from build123d import *

# Parameters (mm, degrees)
SKETCH1_R               = 2.54
BOSS_EXTRUDE1_DEPTH     = 15.24
CUT_EXTRUDE1_DEPTH      = 28.358513503
SKETCH3_W               = 3.302
SKETCH3_H               = 15.39875
CUT_EXTRUDE2_DEPTH      = 26.630137107
CUT_EXTRUDE2_DEPTH_BACK = 26.630137107
SKETCH5_R               = 5.9055
SKETCH5_R_2             = 2.54
BOSS_EXTRUDE2_DEPTH     = 3.81
CUT_EXTRUDE3_DEPTH      = 3.81
FILLET1_R               = 1.27


with BuildPart() as part:
    # Sketch1 → Boss-Extrude1 (new body)
    with BuildSketch(Plane(origin=(0, 0, 0), x_dir=(0, 0, -1), z_dir=(1, 0, 0))):
        with BuildLine():
            Line((-6.35, 0), (-4.6736, 0))
            Line((-4.6736, 0), (-4.6736, -15.7))
            Line((-4.6736, -15.7), (-1.6256, -15.7))
            Line((-1.6256, -15.7), (-1.6256, 0))
            Line((-1.6256, 0), (1.6256, 0))
            Line((1.6256, 0), (1.6256, -15.7))
            Line((1.6256, -15.7), (4.6736, -15.7))
            Line((4.6736, -15.7), (4.6736, 0))
            Line((4.6736, 0), (6.35, 0))
            Line((6.35, 0), (6.35, 6.319735583))
            ThreePointArc((6.35, 6.319735583), (6.479041034, 7.59337978), (6.86091954, 8.815259453))
            ThreePointArc((6.86091954, 8.815259453), (0, 19.20875), (-6.86091954, 8.815259453))
            ThreePointArc((-6.86091954, 8.815259453), (-6.479041034, 7.59337978), (-6.35, 6.319735583))
            Line((-6.35, 6.319735583), (-6.35, 0))
        make_face()
        with Locations((0, 11.7475)):
            Circle(SKETCH1_R, mode=Mode.SUBTRACT)
    extrude(amount=-BOSS_EXTRUDE1_DEPTH)

    # Sketch2 → Cut-Extrude1 (cut, through all)
    with BuildSketch(Plane.XY.offset(4.6736)):
        with BuildLine():
            ThreePointArc((-5.08, -8.08), (-5.823948776, -6.283948776), (-7.62, -5.54))
            Line((-7.62, -5.54), (-7.62, -10.62))
            ThreePointArc((-7.62, -10.62), (-5.823948776, -9.876051224), (-5.08, -8.08))
        make_face()
        with BuildLine():
            Line((-7.62, -10.62), (-7.62, -5.54))
            ThreePointArc((-7.62, -5.54), (-10.16, -8.08), (-7.62, -10.62))
        make_face()
        with BuildLine():
            ThreePointArc((-7.62, -15.7), (-13.008153673, -13.468153673), (-15.24, -8.08))
            Line((-15.24, -8.08), (-15.24, -15.7))
            Line((-15.24, -15.7), (-7.62, -15.7))
        make_face()
        with BuildLine():
            Line((0, -15.7), (0, -8.08))
            ThreePointArc((0, -8.08), (-2.231846327, -13.468153673), (-7.62, -15.7))
            Line((-7.62, -15.7), (0, -15.7))
        make_face()
    extrude(amount=-CUT_EXTRUDE1_DEPTH, mode=Mode.SUBTRACT)

    # Sketch3 → Cut-Extrude2 (cut, two sides)
    with BuildSketch(Plane.XY) as cut_extrude2_sk:
        with Locations((-4.318, 11.509375)):
            Rectangle(SKETCH3_W, SKETCH3_H)
        with Locations((-10.922, 11.509375)):
            Rectangle(SKETCH3_W, SKETCH3_H)
    extrude(amount=CUT_EXTRUDE2_DEPTH, mode=Mode.SUBTRACT)
    extrude(cut_extrude2_sk.sketch, amount=-CUT_EXTRUDE2_DEPTH_BACK, mode=Mode.SUBTRACT)

    # Sketch5 → Boss-Extrude2 (add)
    with BuildSketch(Plane(origin=(0, 0, 0), x_dir=(0, 0, -1), z_dir=(1, 0, 0))):
        with Locations(Location((0, 11.7475, 0), (0, 0, 180))):
            Circle(SKETCH5_R)
        with Locations((0, 11.7475)):
            Circle(SKETCH5_R_2, mode=Mode.SUBTRACT)
    extrude(amount=BOSS_EXTRUDE2_DEPTH)

    # Sketch6 → Cut-Extrude3 (cut)
    with BuildSketch(Plane(origin=(3.81, 0, 0), x_dir=(0, 0, -1), z_dir=(1, 0, 0))):
        Polygon((0, 16.322885413), (-3.9624, 14.035192707), (-3.9624, 9.459807293), (0, 7.172114587), (3.9624, 9.459807293), (3.9624, 14.035192707), align=None)
    extrude(amount=-CUT_EXTRUDE3_DEPTH, mode=Mode.SUBTRACT)

    # Fillet1
    fillet1_edges = [part.edges().sort_by_distance(p)[0] for p in [
        (0, 11.7475, -5.9055),
        (3.81, 11.7475, -5.9055),
        (-15.24, 3.159867792, -6.35),
        (-15.24, 7.59337978, -6.479041034),
        (-15.24, 3.159867792, 6.35),
        (-15.24, 19.20875, 0),
        (-15.24, 7.59337978, 6.479041034),
    ]]
    fillet(fillet1_edges, radius=FILLET1_R)


solid = part.part
Check sheet for the modelled part. Datum: model origin and axes. Units: mm. A direction names the side the tool comes from. Coordinates: 2 decimals unless noted, no trailing zeros. Loops run counter-clockwise (first coordinate to the right, second up) from the corner with the lowest first, then second, coordinate; pieces in that order, holes last. Notation, with made-up numbers: (36.5, 18.5) -> (74.5, 18.5) arc R11 cw to (74.5, 38.5) -> close; hole circle Ø11 at (-36.5, 27.5). An arc over 180 degrees is marked (long way). Write item = value, one per line. Start each with the question number.
1. Section check A-A on x = -2. Record the cut outline in (y, z), then the cut area to 3 significant figures.
2. Material ranges on line 1 (X direction, y = 13.5, z = -3); line 2 (X direction, y = 14.5, z = -3.5); line 3 (Y direction, x = -1.55, z = 0), recorded low to high.
3. Draft check along Y on faces 6 (the flat face through (-7, 3, 6.35)), 7 (the flat face through (1.93, 8.3, -1.95)), 8 (the cylindrical face through (-13.262, 7.576, -6.475)). Enter one of: released by +Y, released by -Y, zero draft, split by the parting line, or undercut.
4. Tool access check on faces 1 (the flat face through (-8, 0, 6)), 2 (the flat face through (-7, 2, -6.35)), 3 (the cylindrical face through (1.896, 5.892, -0.769)), 4 (the flat face through (-5.8, -6, -1.626)), 5 (the flat face through (-11, 3.81, 0)). Record the directions out of +Z, -Z, +X, -X, +Y, -Y that give a thin tool (end or side, any length) a straight path to the whole face; none if there is none.
5. Section check B-B on y = 1. Record the cut outline in (x, z).
6. Section check C-C on z = 2. Give the number of separate pieces and of enclosed holes in the cut face, then the cut area to 3 significant figures.
7. Depth check by flat-ended pin: P1, Ø7.5, axis at x = -5, y = -11.5, coming from the -Z side; P2, Ø1.1, axis at x = 2, y = 11, coming from the +Z side; P3, Ø4, axis at x = -12, y = -10, coming from the +Z side; P4, Ø4.5, axis at y = 14, z = 3, coming from the +X side. Enter the tip coordinate at first touch or a pass-through.
Responses:
q1.outline = (-13.23, -4.67) -> (0, -4.67) -> (0, -6.35) -> (6.32, -6.35) arc R6.35 cw to (8.82, -6.86) arc R7.46 ccw (long way) to (8.82, 6.86) arc R6.35 cw to (6.32, 6.35) -> (0, 6.35) -> (0, 4.67) -> (-13.23, 4.67) -> (-13.23, 1.63) -> (0, 1.63) -> (0, -1.63) -> (-13.23, -1.63) -> close; hole circle Ø5.08 at (11.75, 0)
q1.area = 303 mm2
q2.line_1 = -15.24 to -12.57, -9.27 to -5.97, -2.67 to 0
q2.line_2 = -15.24 to -12.57, -9.27 to -5.97, -2.67 to 3.81
q2.line_3 = 0 to 9.21, 14.29 to 19.21
q3.face_6 = zero draft
q3.face_7 = undercut
q3.face_8 = released by -Y
q4.face_1 = +Z, +X, -X, -Y
q4.face_2 = -Z, +X, -X, -Y
q4.face_3 = +X
q4.face_4 = +X, -X, -Y
q4.face_5 = +Z, -Z, +Y
q5.outline = (-15.24, -5.08) arc R1.27 ccw to (-13.97, -6.35) -> (0, -6.35) -> (0, 6.35) -> (-13.97, 6.35) arc R1.27 ccw to (-15.24, 5.08) -> close
q6.separate_pieces = 4
q6.enclosed_holes = 1
q6.area = 372 mm2
q7.P1 = -4.67
q7.P2 = 5.9
q7.P3 = 4.67
q7.P4 = 3.81
